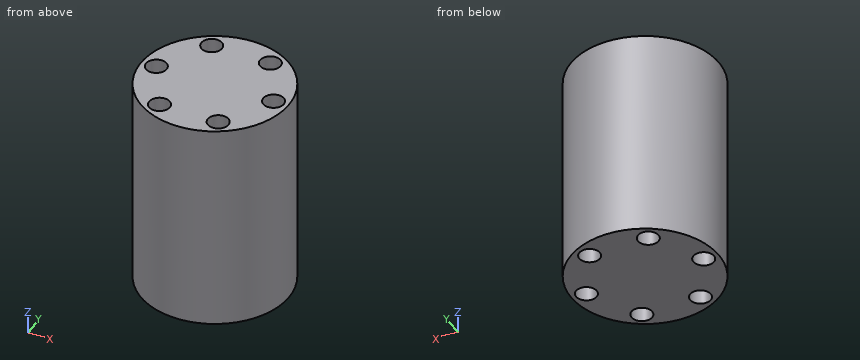
from build123d import *

# Parameters (mm, degrees)
SKETCH1_R           = 15
BOSS_EXTRUDE1_DEPTH = 21.5
SKETCH2_R           = 2.1
CUT_EXTRUDE1_DEPTH  = 48.947888379


with BuildPart() as part:
    # Sketch1 → Boss-Extrude1 (new, symmetric)
    with BuildSketch(Plane.XY):
        Circle(SKETCH1_R)
    extrude(amount=BOSS_EXTRUDE1_DEPTH, both=True)

    # Sketch2 → Cut-Extrude1 (cut, through all)
    with BuildSketch(Plane.XY.offset(21.5)):
        with Locations((-12, 0)):
            Circle(SKETCH2_R)
        with Locations((-6, 10.392304845)):
            Circle(SKETCH2_R)
        with Locations((6, 10.392304845)):
            Circle(SKETCH2_R)
        with Locations((12, 0)):
            Circle(SKETCH2_R)
        with Locations((6, -10.392304845)):
            Circle(SKETCH2_R)
        with Locations((-6, -10.392304845)):
            Circle(SKETCH2_R)
    extrude(amount=-CUT_EXTRUDE1_DEPTH, mode=Mode.SUBTRACT)


solid = part.part
Build history of the part. All positions in model axes, mm. Coordinates: 2 decimals unless noted, no trailing zeros. Order: outer loops, then holes, each group sorted by start corner. A loop starts at its lowest first (then second) coordinate and runs counter-clockwise, first axis right, second up. Notation, with made-up numbers: (75, -20.75) - (102, -20.75) arc R5 cw to (102, -11.75) - close; hole circle Ø7 at (-19.5, 69). An arc over 180 degrees is marked (long way). Write item = value, one per line. Start each with the question number.
1) Saw through at D-D on z = 7. Write the cut outline in (x, y).
2) Saw through at C-C on x = 6. Write the cut outline in (y, z).
3) Saw through at A-A on x = 12. Write the cut outline in (y, z).
4) Flat gauge pins, fed straight in: pin 1 Ø6 at (x, z) = (-4, -1) entering from +Y; pin 2 Ø6 at (x, z) = (-7.5, 1.5) entering from +Y; pin 3 Ø1.5 at (y, z) = (-2, -3.5) entering from +X. Where does each tip first touch, or does it go through?
5) Wall check: line 1 along X through (y, z) = (9, 14); line 2 along X through (y, z) = (1, -14.5); line 3 along Y through (x, z) = (6, -13). Give the ranges that are in metal, low to high. Write a range as from..to.
6) Saw through at B-B on y = 11. Write the cut outline in (x, z), then the cut area to 3 significant figures.
From the geometry:
q1.outline = circle Ø30 at (0, 0); hole circle Ø4.2 at (-12, 0); hole circle Ø4.2 at (-6, -10.39); hole circle Ø4.2 at (-6, 10.39); hole circle Ø4.2 at (6, -10.39); hole circle Ø4.2 at (6, 10.39); hole circle Ø4.2 at (12, 0)
q2.outline = (-13.75, -21.5) - (-12.49, -21.5) - (-12.49, 21.5) - (-13.75, 21.5) - close; (-8.29, -21.5) - (8.29, -21.5) - (8.29, 21.5) - (-8.29, 21.5) - close; (12.49, -21.5) - (13.75, -21.5) - (13.75, 21.5) - (12.49, 21.5) - close
q3.outline = (-9, -21.5) - (-2.1, -21.5) - (-2.1, 21.5) - (-9, 21.5) - close; (2.1, -21.5) - (9, -21.5) - (9, 21.5) - (2.1, 21.5) - close
q4.pin_1 = 14.97
q4.pin_2 = 14.31
q4.pin_3 = 14.95
q5.line_1 = -12..-7.57, -4.43..4.43, 7.57..12
q5.line_2 = -14.97..-13.85, -10.15..10.15, 13.85..14.97
q5.line_3 = -13.75..-12.49, -8.29..8.29, 12.49..13.75
q6.outline = (-10.2, -21.5) - (-8.01, -21.5) - (-8.01, 21.5) - (-10.2, 21.5) - close; (-3.99, -21.5) - (3.99, -21.5) - (3.99, 21.5) - (-3.99, 21.5) - close; (8.01, -21.5) - (10.2, -21.5) - (10.2, 21.5) - (8.01, 21.5) - close
q6.area = 531 mm^2
